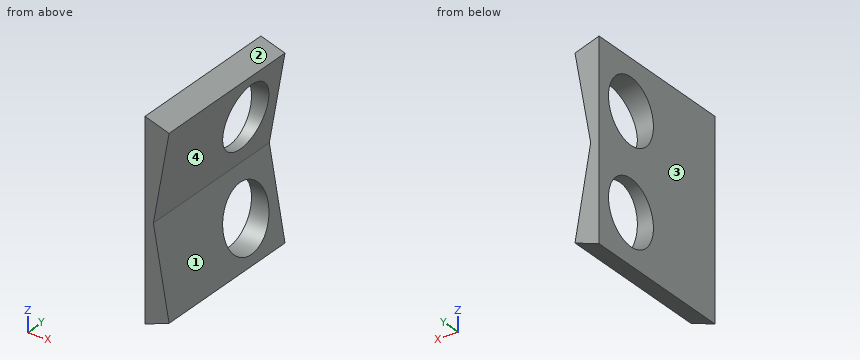
```python
from build123d import *

# Parameters (mm, degrees)
BOSS_EXTRUDE2_DEPTH = 40
CUT_EXTRUDE1_REACH  = 48.78
SKETCH4_R           = 7.75


with BuildPart() as part:
    # Sketch3 → Boss-Extrude2 (new body)
    with BuildSketch(Plane(origin=(0, 0, 0), x_dir=(1, 0, 0), z_dir=(0, 1, 0))):
        Polygon((0, -23.54499856), (5.828357437, -21.536716606), (2.030853224, 0), (5.828357437, 21.536716606), (0, 23.54499856), align=None)
    extrude(amount=BOSS_EXTRUDE2_DEPTH)

    # Sketch4 → Cut-Extrude1 (cut, up to next)
    with BuildSketch(Plane.ZY, mode=Mode.PRIVATE) as cut_extrude1_sk1:
        with Locations((-11.5, 29)):
            Circle(SKETCH4_R)
    cut_extrude1_tool1 = extrude(cut_extrude1_sk1.sketch, amount=-CUT_EXTRUDE1_REACH, mode=Mode.PRIVATE) & part.part
    # Sketch4 → Cut-Extrude1 (cut, up to next)
    with BuildSketch(Plane.ZY, mode=Mode.PRIVATE) as cut_extrude1_sk2:
        with Locations((11.5, 29)):
            Circle(SKETCH4_R)
    cut_extrude1_tool2 = extrude(cut_extrude1_sk2.sketch, amount=-CUT_EXTRUDE1_REACH, mode=Mode.PRIVATE) & part.part
    add(cut_extrude1_tool1.solids().sort_by_distance((0, 29, -11.5))[0], mode=Mode.SUBTRACT)
    add(cut_extrude1_tool2.solids().sort_by_distance((0, 29, 11.5))[0], mode=Mode.SUBTRACT)


solid = part.part
```
Part model, mm, in its own coordinate system. Face numbers are marked on the shaded views. Coordinates: 2 decimals unless noted, no trailing zeros. Loops run counter-clockwise (first coordinate to the right, second up) from the corner with the lowest first, then second, coordinate; pieces in that order, holes last. Notation, with made-up numbers: (76.25, 84) - (128.25, 84) arc R27 cw to (128.25, 121) - close; hole circle Ø4 at (68, 13.5). An arc over 180 degrees is marked (long way). Write item = value, one per line. Start each with the question number.
Item 1: Cut at A-A, the plane y = 25. Give the cut face in (x, z) (3 decimals), and give its area (3 significant figures).
Item 2: Wall check: L1, parallel to Y at x = 1.2, z = 11.5; L2, parallel to Z at x = 0.45, y = 23.5; L3, parallel to Z at x = 0.75, y = 28. Give the ranges that are in metal, low to high. Write a range as from..to.
Item 3: Mould opens along Z. For the marked faces 1, 2, 3 and 4 say: released by +Z, released by -Z, zero draft, split by the parting line, or undercut.
Item 4: Cut at B-B, the plane z = -11.5. Give the cut face in (x, y).
Item 5: Cut at D-D, the plane y = 19. Give the cut face in (x, z) (3 decimals), and give its area (3 significant figures).
Item 6: Cut at C-C, the plane x = 1.2. Give the cut face in (y, z), and give its area (3 significant figures).
The answers:
q1.outline = (0, -23.545) - (5.828, -21.537) - (5.229, -18.138) - (0, -18.138) - close; (0, -4.862) - (2.888, -4.862) - (2.031, 0) - (2.888, 4.862) - (0, 4.862) - close; (0, 18.138) - (5.229, 18.138) - (5.828, 21.537) - (0, 23.545) - close
q1.area = 73.2 mm2
q2.L1 = 0..21.25, 36.75..40
q2.L2 = -23.39..-16.96, -6.04..6.04, 16.96..23.39
q2.L3 = -23.29..-19.19, -3.81..3.81, 19.19..23.29
q3.face_1 = undercut
q3.face_2 = released by +Z
q3.face_3 = zero draft
q3.face_4 = undercut
q4.outline = (0, 0) - (4.06, 0) - (4.06, 21.25) - (0, 21.25) - close; (0, 36.75) - (4.06, 36.75) - (4.06, 40) - (0, 40) - close
q5.outline = (0, -23.545) - (5.828, -21.537) - (2.031, 0) - (5.828, 21.537) - (0, 23.545) - close
q5.area = 181 mm2
q6.outline = (0, -23.13) - (40, -23.13) - (40, 23.13) - (0, 23.13) - close; hole circle Ø15.5 at (29, -11.5); hole circle Ø15.5 at (29, 11.5)
q6.area = 1,470 mm2
